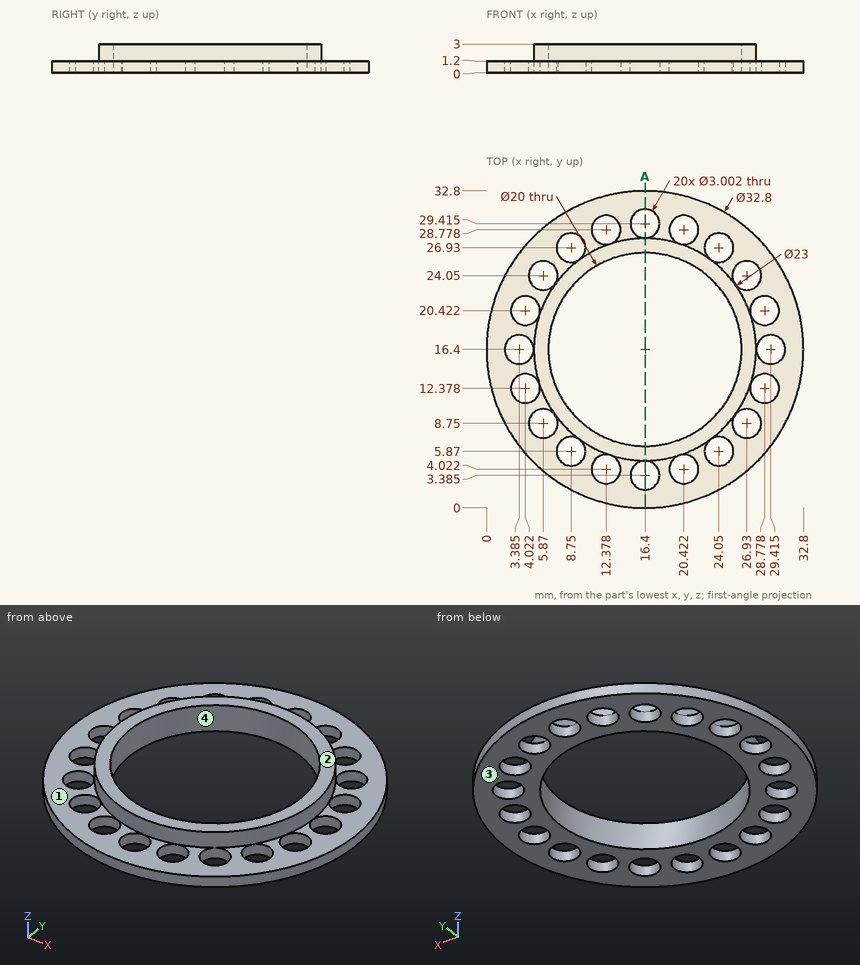
Can you work these out from the drawing? Everything is in mm from the part's minimum corner. A direction names the side the tool comes from. Give positions to 0.01 mm unless a question says otherwise; leave off trailing zeros. Return JSON: item names as keys, results as strings.
1. For pin 1 Ø2.5 at (x, y) = (12.38, 28.78) entering from -Z; pin 2 Ø1.5 at (y, z) = (25.5, 0.5) entering from -X (1 decimal), each with a flat end and sliding along its axis, tell me the tip position at first contact or that it passes through.
Answer list:
{"pin 1": "passes through", "pin 2": "stops at x = 2.3"}
2. Imagine slicing it at A-A on x = 16.4. Give the number of separate pieces and of enclosed holes in the cut face.
Answer list:
{"separate pieces": "4", "enclosed holes": "0"}
3. On a 3-axis mill with a long thin cutter (end or side, diameter ignored), from which of +Z, -Z, +X, -X, +Y, -Y can I reach the whole of each face in a straight line? I mean the marked faces 1 and 2. Say none if no direction works.
Answer list:
{"face 1": "+Z", "face 2": "+Z, +X, -X, +Y, -Y"}
4. Thinking about a two-plate mould opening in Y: for the marked faces 3 and 4, which applies, pulls with the +Y half, pulls with the -Y half, needs draft (parallel to the pull), parting line crosses it, or undercut?
Answer list:
{"face 3": "needs draft", "face 4": "undercut"}
5. I need wall thicknesses on line 1 (Y direction, x = 4.5, z = 0.95) (1 decimal); line 2 (X direction, y = 4, z = 1) (1 decimal); line 3 (Y direction, x = 9.5, z = 0.45). Which ranges of each line are inside material? Lowest first, please. Write a range as from..to.
Answer list:
{"line 1": "y = 5.1..8.1, 9.4..11, 13.8..15.4, 17.4..19, 21.8..23.4, 24.7..27.7", "line 2": "x = 5.7..10.9, 13.9..15, 17.8..18.9, 21.9..27.1", "line 3": "y = 1.52..4.57, 7.17..9.16, 23.64..25.63, 28.23..31.28"}
